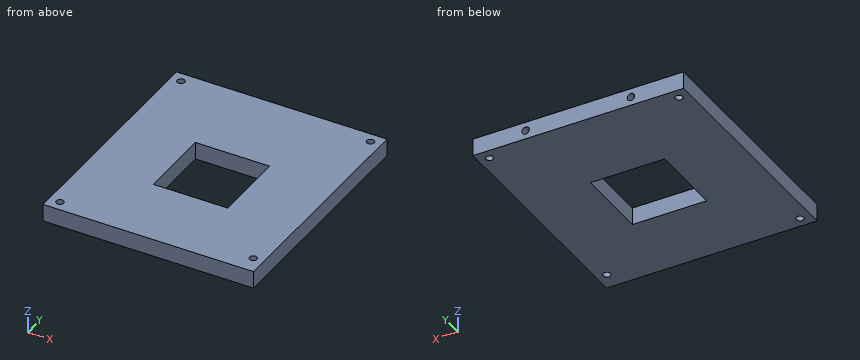
from build123d import *

# Parameters (mm, degrees)
SKETCH1_W           = 85
SKETCH1_H           = 95
BOSS_EXTRUDE1_DEPTH = 7
SKETCH2_W           = 30
SKETCH2_H           = 30
CUT_EXTRUDE1_DEPTH  = 7
SKETCH4_R           = 1.5
CUT_EXTRUDE2_DEPTH  = 5
SKETCH6_R           = 1.5
CUT_EXTRUDE3_DEPTH  = 8


with BuildPart() as part:
    # Sketch1 → Boss-Extrude1 (new body)
    with BuildSketch(Plane.XY):
        with Locations((42.5, 47.5)):
            Rectangle(SKETCH1_W, SKETCH1_H)
    extrude(amount=BOSS_EXTRUDE1_DEPTH)

    # Sketch2 → Cut-Extrude1 (cut)
    with BuildSketch(Plane.XY.offset(7)):
        with Locations((42.5, 45)):
            Rectangle(SKETCH2_W, SKETCH2_H)
    extrude(amount=-CUT_EXTRUDE1_DEPTH, mode=Mode.SUBTRACT)

    # Sketch4 → Cut-Extrude2 (cut)
    with BuildSketch(Plane(origin=(0, 95, 0), x_dir=(1, 0, 0), z_dir=(0, 1, 0))):
        with Locations((21.25, -3.5)):
            Circle(SKETCH4_R)
        with Locations((63.75, -3.5)):
            Circle(SKETCH4_R)
    extrude(amount=-CUT_EXTRUDE2_DEPTH, mode=Mode.SUBTRACT)

    # Sketch6 → Cut-Extrude3 (cut)
    with BuildSketch(Plane(origin=(0, 0, 0), x_dir=(-1, 0, 0), z_dir=(0, 0, -1))):
        with Locations((-80.75, 90.75)):
            Circle(SKETCH6_R)
        with Locations((-4.25, 90.75)):
            Circle(SKETCH6_R)
        with Locations((-4.45, 4.25)):
            Circle(SKETCH6_R)
        with Locations((-80.75, 7.25)):
            Circle(SKETCH6_R)
    extrude(amount=-CUT_EXTRUDE3_DEPTH, mode=Mode.SUBTRACT)


solid = part.part
Check sheet for the modelled part. Datum: model origin and axes. Units: mm. Round coordinates to 2 decimals unless told otherwise and drop trailing zeros. Order: outer loops, then holes, each group sorted by start corner. A loop starts at its lowest first (then second) coordinate and runs counter-clockwise, first axis right, second up. Notation, with made-up numbers: M -37,1.25 L -4,1.25 A23 ccw -4,25.25 Z; hole C 39.5,76.25 d9. An arc over 180 degrees is marked long. One line per item, written item: value. Start each with the question number.
1. Section check B-B on y = 37. Enter the section's corners in (x, z).
2. Scan lines: line 1 along X through (y, z) = (90.75, 3.5); line 2 along Y through (x, z) = (4.25, 2); line 3 along X through (y, z) = (46.5, 1). Record each from-to range of solid material in increasing order.
3. Gauge pin test, flat ends, axial feed: P1, Ø2.5, axis at x = 80.75, y = 90.75, coming from the +Z side; P2, Ø1.5, axis at x = 21.5, z = 4, coming from the +Y side. Record the tip position at first contact, or that the pin passes through.
4. Section check C-C on x = 4.25. Enter the section's corners in (y, z).
5. Section check A-A on x = 50.5. Enter the section's corners in (y, z), and give its area (3 significant figures).
Results found:
1. outline: M 0,0 L 27.5,0 L 27.5,7 L 0,7 Z; M 57.5,0 L 85,0 L 85,7 L 57.5,7 Z
2. line 1: 0 to 2.75, 5.75 to 19.75, 22.75 to 62.25, 65.25 to 79.25, 82.25 to 85
2. line 2: 0 to 2.76, 5.74 to 89.25, 92.25 to 95
2. line 3: 0 to 27.5, 57.5 to 85
3. P1: through
3. P2: y = 90
4. outline: M 0,0 L 2.76,0 L 2.76,7 L 0,7 Z; M 5.74,0 L 89.25,0 L 89.25,7 L 5.74,7 Z; M 92.25,0 L 95,0 L 95,7 L 92.25,7 Z
5. outline: M 0,0 L 30,0 L 30,7 L 0,7 Z; M 60,0 L 95,0 L 95,7 L 60,7 Z
5. area: 455 mm^2
